Work out the finished part from the listing and answer in its coordinate system (mm). Face numbers are marked on the shaded views. A direction names the side the tool comes from. Coordinates: 2 decimals unless noted, no trailing zeros. Order: outer loops, then holes, each group sorted by start corner. A loop starts at its lowest first (then second) coordinate and runs counter-clockwise, first axis right, second up. Notation, with made-up numbers: (0.25, 46) - (48.25, 46) arc R22 cw to (48.25, 73) - close; hole circle Ø5 at (3.25, -10). An arc over 180 degrees is marked (long way). Answer as a JSON object with one key per item and string values. Group by question number.
1) The mould has two halves that part along Z. Classify the marked faces 5, 6, 7 and 8: released by +Z, released by -Z, zero draft, split by the parting line, or undercut.
2) Section D-D (x = 37) is taken. Give the vertices of the cut face in (y, z), plus the area to 3 significant figures.
3) Section C-C (z = 5.25) is taken. Give the vertices of the cut face in (x, y), plus the area to 3 significant figures.
4) Section B-B (x = -11.5) is taken. Give the vertices of the cut face in (y, z).
5) Each of these flat-tipped pins is pushed along its axis until it touches: P1, Ø2, axis at x = -14.5, z = -13.5, coming from the +Y side; P2, Ø10, axis at y = 23, z = -4.5, coming from the -X side; P3, Ø3, axis at x = 33.5, z = -4, coming from the +Y side; P4, Ø5, axis at x = -40, z = -2, coming from the -Y side. Where does it stop, or does it pass through?
6) A tool of negligible diameter and unlimited length cuts with its end or side. For the marked faces 1, 2, 3 and 4, from which of +Z, -Z, +X, -X, +Y, -Y can it reach the whole face along a straight path? Write none if from no direction.
7) Section A-A (z = -2.5) is taken. Give the vertices of the cut face in (x, y), plus the area to 3 significant figures.
8) Find the intervals of material crossed by line 1 along Y through (x, z) = (-34, 4.5); line 2 along Y through (x, z) = (-3, 6.5); line 3 along Y through (x, z) = (20, 0.5), in increasing order.
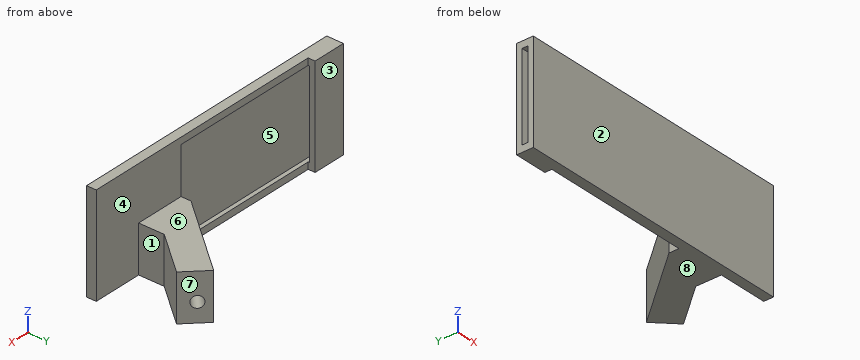
from build123d import *

# Parameters (mm, degrees)
SKETCH1_W           = 85
SKETCH1_H           = 30
BOSS_EXTRUDE1_DEPTH = 5
SKETCH2_W           = 26
SKETCH2_H           = 1.7
CUT_EXTRUDE1_DEPTH  = 55
SKETCH3_W           = 75
SKETCH3_H           = 30
CUT_EXTRUDE2_DEPTH  = 2.1
BOSS_EXTRUDE5_DEPTH = 14


with BuildPart() as part:
    # Sketch1 → Boss-Extrude1 (new body)
    with BuildSketch(Plane(origin=(0, 0, 0), x_dir=(1, 0, 0), z_dir=(0, 1, 0))):
        Rectangle(SKETCH1_W, SKETCH1_H)
    extrude(amount=BOSS_EXTRUDE1_DEPTH)

    # Sketch2 → Cut-Extrude1 (cut)
    with BuildSketch(Plane.ZY.offset(42.5)):
        with Locations((0, 2.5)):
            Rectangle(SKETCH2_W, SKETCH2_H)
    extrude(amount=-CUT_EXTRUDE1_DEPTH, mode=Mode.SUBTRACT)

    # Sketch3 → Cut-Extrude2 (cut)
    with BuildSketch(Plane(origin=(0, 5, 0), x_dir=(1, 0, 0), z_dir=(0, 1, 0))):
        with Locations((5, 0)):
            Rectangle(SKETCH3_W, SKETCH3_H)
    extrude(amount=-CUT_EXTRUDE2_DEPTH, mode=Mode.SUBTRACT)

    # Sketch10 → Boss-Extrude5 (add)
    with BuildSketch(Plane(origin=(0, 0, -15), x_dir=(-1, 0, 0), z_dir=(0, 0, -1))):
        Polygon((-27.5, 2.9), (-12.5, 2.9), (-12.5, 5.9), (-32.105022095, 29.264355515), (-38.115429736, 23.253947875), (-27.5, 10.552651361), align=None)
    extrude(amount=-BOSS_EXTRUDE5_DEPTH)

    # Sketch14 → Cut-Revolve5 (revolve, cut)
    with BuildSketch(Plane(origin=(4.05, -4.05, 0), x_dir=(0, 0, 1), z_dir=(-0.7071067811865432, 0.7071067811865518, 0)), mode=Mode.PRIVATE) as cut_revolve5_sk:
        Polygon((-9.8, 10.005560954), (-9.2, 10.005560954), (-9.3, 43.905413461), (-11.05, 43.905413461), align=None)
    revolve(cut_revolve5_sk.sketch.rotate(Axis((11.125, 3.025, -9.2), (0.7071037046891342, 0.7071037046891259, -0.0029498525073746134)), 89.830986391), axis=Axis((11.125, 3.025, -9.2), (0.7071037046891342, 0.7071037046891259, -0.0029498525073746134)), mode=Mode.SUBTRACT)


solid = part.part
Report:
{
 "1": {"face 5": "undercut", "face 6": "released by +Z", "face 7": "zero draft", "face 8": "released by -Z"},
 "2": {"outline": "(0, -15) - (2.9, -15) - (2.9, 15) - (0, 15) - close; (21.92, -15) - (24.37, -15) - (24.37, -1) - (21.92, -1) - close", "area": "121 mm²"},
 "3": {"outline": "(-42.5, 0) - (42.5, 0) - (42.5, 2.9) - (12.5, 2.9) - (12.5, 1.65) - (-42.5, 1.65) - close; (-42.5, 3.35) - (-32.5, 3.35) - (-32.5, 5) - (-42.5, 5) - close", "area": "194 mm²"},
 "4": {"outline": "(0, -15) - (2.9, -15) - (2.9, -13) - (1.65, -13) - (1.65, 13) - (2.9, 13) - (2.9, 15) - (0, 15) - close"},
 "5": {"P1": "stops at y = 2.9", "P2": "stops at x = 22.65", "P3": "stops at y = 29.26", "P4": "stops at y = 0"},
 "6": {"face 1": "+Z, -Z, +X", "face 2": "+Z, -Z, +X, -X, -Y", "face 3": "+Z, -Z, -X, +Y", "face 4": "+Z, +X"},
 "7": {"outline": "(-42.5, 0) - (42.5, 0) - (42.5, 2.9) - (27.5, 2.9) - (27.5, 10.55) - (38.12, 23.25) - (32.11, 29.26) - (12.5, 5.9) - (12.5, 1.65) - (-42.5, 1.65) - close; (-42.5, 3.35) - (-32.5, 3.35) - (-32.5, 5) - (-42.5, 5) - close", "area": "474 mm²"},
 "8": {"line 1": "y = 0 to 1.65, 3.35 to 5", "line 2": "y = 0 to 1.65", "line 3": "y = 0 to 2.9"}
}
